The model under review builds one solid part; all positions refer to its coordinate system, in mm. A direction names the side the tool comes from. Coordinates: 2 decimals unless noted, no trailing zeros. Loops run counter-clockwise (first coordinate to the right, second up) from the corner with the lowest first, then second, coordinate; pieces in that order, holes last. Notation, with made-up numbers: (70, -33) -> (101, -33) arc R18 ccw to (101, -12) -> close; hole circle Ø4 at (-4, 0). An arc over 180 degrees is marked (long way). One line per question, with ' | ' between items. Start each with the question number.
from build123d import *

# Parameters (mm, degrees)
F0_R        = 4.7625
F1_DEPTH    = 6.35
F2_T1_DEPTH = 6.35
F2_T3_DEPTH = 129.3172212421
F3_R        = 50.8


# Not quite as in the source:
# - a fillet or chamfer that OpenCascade refuses, or shapes differently, is made with other operations: its cross-section is extruded or revolved along the edge and cut away or added


with BuildPart() as f1:
    # F0 (on Top) → F1 (new body)
    with BuildSketch(Plane.XY):
        with BuildLine():
            Line((25.4, -63.5), (25.4, 23.0659139254))
            Line((25.4, 23.0659139254), (-6.3346226919, 59.1827919466))
            ThreePointArc((-6.3346226919, 59.1827919466), (-24.2577919466, 60.3403773081), (-25.4153773081, 42.4172080534))
            Line((-25.4153773081, 42.4172080534), (0, 13.4922042489))
            Line((0, 13.4922042489), (0, 0))
            Line((0, 0), (6.35, 0))
            Line((6.35, 0), (6.35, -63.5))
            Line((6.35, -63.5), (25.4, -63.5))
        make_face()
        with Locations((-15.875, 50.8)):
            Circle(F0_R, mode=Mode.SUBTRACT)
    extrude(amount=F1_DEPTH)

    # F2: fillet of radius 25.4 on 2 edges, made by hand

    # F2_s2 → F2_t1 (join)
    with BuildSketch(Plane.XY):
        with BuildLine():
            ThreePointArc((-6.3192453838, 20.6840784656), (-1.6322574983, 12.8769775006), (0, 3.9184945725))
            Line((0, 3.9184945725), (0, 13.4922042489))
            Line((0, 13.4922042489), (-6.3192453838, 20.6840784656))
        make_face()
    extrude(amount=F2_T1_DEPTH)

    # F2_s4 → F2_t3 (cut)
    with BuildSketch(Plane.XY.offset(-61.483610621)):
        with BuildLine():
            ThreePointArc((6.35, -63.5), (20.0804631421, -54.4608156183), (25.4, -38.9065557516))
            Line((25.4, -38.9065557516), (25.4, -63.5))
            Line((25.4, -63.5), (6.35, -63.5))
        make_face()
    extrude(amount=F2_T3_DEPTH, mode=Mode.SUBTRACT)

    # F3
    f3_edges = [f1.edges().sort_by_distance(p)[0] for p in [
        (25.4, 23.065914, 3.175),
    ]]
    fillet(f3_edges, radius=F3_R)


solid = f1.part
1) Wall thickness on L1, parallel to Y at x = -5, z = 4.25; L2, parallel to Y at x = 15, z = 3.75; L3, parallel to X at y = -13, z = 4.25: over which ranges is each line inside the solid? List them lowest first.
2) Machinability: for faces 4 (the face through (0, 2, 3)), 5 (the face through (4, 15, 6.35)), which of the approach directions +Z, -Z, +X, -X, +Y, -Y give a long, thin tool a straight path to every point of the face, cutting with its end or side? Answer none if there is none.
3) Consider section D-D, the plane y = -27. Write out the cut boundary in (x, z).
4) Mouldability with a two-part tool opening along Y and no side actions: class faces 1 (the face through (22.044, 22.075, 3.219)), 2 (the face through (25.4, -18, 3)), 3 (the face through (-19.4, 54, 3.1)) as +Y half, -Y half, draft (parallel to the pull), parting line (faces both ways), or undercut.
5) Consider section B-B, the plane x = -18.5. Write out the cut boundary in (y, z).
6) Insertion check: pin 1 Ø3 at (y, z) = (-41.5, 3.5) entering from -X; pin 2 Ø3 at (x, z) = (3, 4.5) entering from -Y. Each pin has a flat end and moves straight along its axis. Give the tip position at first contact, or say it passes through.
Filled sheet:
1) L1: 19.05 to 57.66 | L2: -59.4 to 34.72 | L3: 6.35 to 25.4
2) face 4: +Z, -Z, -X, -Y | face 5: +Z, +X, -X, +Y, -Y
3) outline: (6.35, 0) -> (25.4, 0) -> (25.4, 6.35) -> (6.35, 6.35) -> close
4) face 1: +Y half | face 2: draft | face 3: undercut
5) outline: (34.55, 0) -> (46.83, 0) -> (46.83, 6.35) -> (34.55, 6.35) -> close; (54.77, 0) -> (63.23, 0) -> (63.23, 6.35) -> (54.77, 6.35) -> close
6) pin 1: x = 6.35 | pin 2: y = 0
